Verification items for the finished model (mm, model axes). Face numbers are marked on the shaded views. Give positions to 0.01 mm unless a question says otherwise; leave off trailing zeros. Loops run counter-clockwise (first coordinate to the right, second up) from the corner with the lowest first, then second, coordinate; pieces in that order, holes last. Notation, with made-up numbers: M 70.5,18.5 L 115.5,18.5 A25 ccw 115.5,36.5 Z; hole C -19,53 d9. An arc over 180 degrees is marked long. Use CSV: the item, a comma, the result in double quotes.
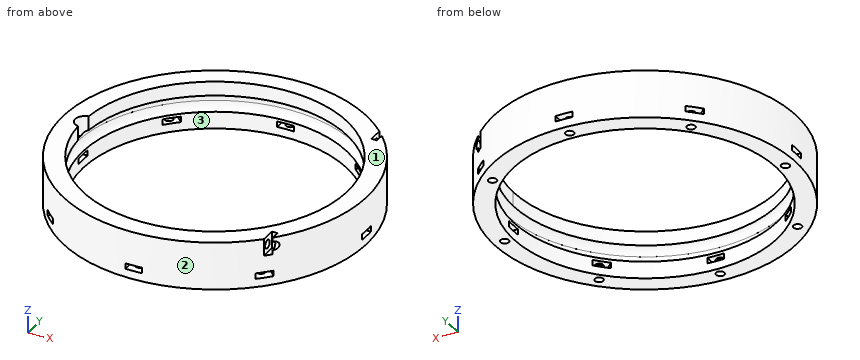
from build123d import *

# Parameters (mm, degrees)
BOX174_W                    = 2
BOX174_H                    = 6
BOX174_DEPTH                = 6
BOX175_W                    = 2
BOX175_H                    = 6
BOX175_DEPTH                = 6
BOX176_W                    = 2
BOX176_H                    = 6
BOX176_DEPTH                = 6
BOX173_W                    = 2
BOX173_H                    = 6
BOX173_DEPTH                = 6
CYLINDER397_R               = 1.5
CYLINDER397_DEPTH           = 100
CYLINDER398_R               = 1.5
CYLINDER398_DEPTH           = 100
CYLINDER395_R               = 1.5
CYLINDER395_DEPTH           = 100
CYLINDER396_R               = 1.5
CYLINDER396_DEPTH           = 100
CYLINDER375_R               = 1.5
CYLINDER375_DEPTH           = 50
CYLINDER375_PLACEMENT_ANGLE = 45
CYLINDER376_R               = 1.5
CYLINDER376_DEPTH           = 50
CYLINDER377_R               = 1.5
CYLINDER377_DEPTH           = 50
CYLINDER377_PLACEMENT_ANGLE = 135
CYLINDER378_R               = 1.5
CYLINDER378_DEPTH           = 50
CYLINDER379_R               = 1.5
CYLINDER379_DEPTH           = 50
CYLINDER379_PLACEMENT_ANGLE = 225
CYLINDER380_R               = 1.5
CYLINDER380_DEPTH           = 50
CYLINDER381_R               = 1.5
CYLINDER381_DEPTH           = 50
CYLINDER381_PLACEMENT_ANGLE = 45
CYLINDER374_R               = 1.5
CYLINDER374_DEPTH           = 50
BOX158_W                    = 8
BOX158_H                    = 6
BOX158_DEPTH                = 2
BOX158_PLACEMENT_ANGLE      = 45
BOX159_W                    = 8
BOX159_H                    = 6
BOX159_DEPTH                = 2
BOX160_W                    = 8
BOX160_H                    = 6
BOX160_DEPTH                = 2
BOX160_PLACEMENT_ANGLE      = 135
BOX161_W                    = 8
BOX161_H                    = 6
BOX161_DEPTH                = 2
BOX162_W                    = 8
BOX162_H                    = 6
BOX162_DEPTH                = 2
BOX162_PLACEMENT_ANGLE      = 225
BOX163_W                    = 8
BOX163_H                    = 6
BOX163_DEPTH                = 2
BOX164_W                    = 8
BOX164_H                    = 6
BOX164_DEPTH                = 2
BOX164_PLACEMENT_ANGLE      = 45
BOX157_W                    = 8
BOX157_H                    = 6
BOX157_DEPTH                = 2
CYLINDER006_R               = 3.5
CYLINDER006_DEPTH           = 10
TORUS004_R                  = 3.1
TUBE002_R                   = 54
TUBE002_R_2                 = 47
TUBE002_DEPTH               = 17


with BuildPart() as krychle174:
    # Box174 → Box174 (new body)
    with BuildSketch(Plane(origin=(32, -54, 22), x_dir=(1, 0, 0), z_dir=(0, 0, 1))):
        with Locations((1, 3)):
            Rectangle(BOX174_W, BOX174_H)
    extrude(amount=BOX174_DEPTH)


with BuildPart() as krychle175:
    # Box175 → Box175 (new body)
    with BuildSketch(Plane(origin=(38, 33, 31), x_dir=(1, 0, 0), z_dir=(0, 0, 1))):
        with Locations((1, 3)):
            Rectangle(BOX175_W, BOX175_H)
    extrude(amount=BOX175_DEPTH)


with BuildPart() as krychle176:
    # Box176 → Box176 (new body)
    with BuildSketch(Plane(origin=(38, -39, 31), x_dir=(1, 0, 0), z_dir=(0, 0, 1))):
        with Locations((1, 3)):
            Rectangle(BOX176_W, BOX176_H)
    extrude(amount=BOX176_DEPTH)


with BuildPart() as compound302:
    # Box173 → Box173 (new body)
    with BuildSketch(Plane(origin=(32, 48, 22), x_dir=(1, 0, 0), z_dir=(0, 0, 1))):
        with Locations((1, 3)):
            Rectangle(BOX173_W, BOX173_H)
    extrude(amount=BOX173_DEPTH)

    # Compound302: union Krychle174, Krychle175, Krychle176
    add(krychle174.part)
    add(krychle175.part)
    add(krychle176.part)


with BuildPart() as obj1:
    # Cylinder397 → Cylinder397 (new body)
    with BuildSketch(Plane(origin=(24, -51, 25), x_dir=(0, 0, -1), z_dir=(1, 0, 0))):
        Circle(CYLINDER397_R)
    extrude(amount=CYLINDER397_DEPTH)


with BuildPart() as obj2:
    # Cylinder398 → Cylinder398 (new body)
    with BuildSketch(Plane(origin=(34, 36, 34), x_dir=(0, 0, -1), z_dir=(1, 0, 0))):
        Circle(CYLINDER398_R)
    extrude(amount=CYLINDER398_DEPTH)


with BuildPart() as obj3:
    # Cylinder395 → Cylinder395 (new body)
    with BuildSketch(Plane(origin=(34, -36, 34), x_dir=(0, 0, -1), z_dir=(1, 0, 0))):
        Circle(CYLINDER395_R)
    extrude(amount=CYLINDER395_DEPTH)


with BuildPart() as compound303:
    # Cylinder396 → Cylinder396 (new body)
    with BuildSketch(Plane(origin=(24, 51, 25), x_dir=(0, 0, -1), z_dir=(1, 0, 0))):
        Circle(CYLINDER396_R)
    extrude(amount=CYLINDER396_DEPTH)

    # Compound303: union obj1, obj2, obj3
    add(obj1.part)
    add(obj2.part)
    add(obj3.part)


with BuildPart() as obj4:
    # Cylinder375 → Cylinder375 (new body)
    with BuildSketch(Plane.XY):
        Circle(CYLINDER375_R)
    extrude(amount=CYLINDER375_DEPTH)


with BuildPart() as obj4_1:
    # Cylinder375 placement: moved
    add(obj4.part.moved(Location((35.355339, 35.355339, -15))).rotate(Axis((35.355339, 35.355339, -15), (0, 0, 1)), CYLINDER375_PLACEMENT_ANGLE))


with BuildPart() as obj5:
    # Cylinder376 → Cylinder376 (new body)
    with BuildSketch(Plane(origin=(0, 50, -15), x_dir=(0, 1, 0), z_dir=(0, 0, 1))):
        Circle(CYLINDER376_R)
    extrude(amount=CYLINDER376_DEPTH)


with BuildPart() as obj6:
    # Cylinder377 → Cylinder377 (new body)
    with BuildSketch(Plane.XY):
        Circle(CYLINDER377_R)
    extrude(amount=CYLINDER377_DEPTH)


with BuildPart() as obj6_1:
    # Cylinder377 placement: moved
    add(obj6.part.moved(Location((-35.355339, 35.355339, -15))).rotate(Axis((-35.355339, 35.355339, -15), (0, 0, 1)), CYLINDER377_PLACEMENT_ANGLE))


with BuildPart() as obj7:
    # Cylinder378 → Cylinder378 (new body)
    with BuildSketch(Plane(origin=(-50, 0, -15), x_dir=(-1, 0, 0), z_dir=(0, 0, 1))):
        Circle(CYLINDER378_R)
    extrude(amount=CYLINDER378_DEPTH)


with BuildPart() as obj8:
    # Cylinder379 → Cylinder379 (new body)
    with BuildSketch(Plane.XY):
        Circle(CYLINDER379_R)
    extrude(amount=CYLINDER379_DEPTH)


with BuildPart() as obj8_1:
    # Cylinder379 placement: moved
    add(obj8.part.moved(Location((-35.355339, -35.355339, -15))).rotate(Axis((-35.355339, -35.355339, -15), (0, 0, 1)), CYLINDER379_PLACEMENT_ANGLE))


with BuildPart() as obj9:
    # Cylinder380 → Cylinder380 (new body)
    with BuildSketch(Plane(origin=(0, -50, -15), x_dir=(0, -1, 0), z_dir=(0, 0, 1))):
        Circle(CYLINDER380_R)
    extrude(amount=CYLINDER380_DEPTH)


with BuildPart() as obj10:
    # Cylinder381 → Cylinder381 (new body)
    with BuildSketch(Plane.XY):
        Circle(CYLINDER381_R)
    extrude(amount=CYLINDER381_DEPTH)


with BuildPart() as obj10_1:
    # Cylinder381 placement: moved
    add(obj10.part.moved(Location((35.355339, -35.355339, -15))).rotate(Axis((35.355339, -35.355339, -15), (0, 0, -1)), CYLINDER381_PLACEMENT_ANGLE))


with BuildPart() as compound298:
    # Cylinder374 → Cylinder374 (new body)
    with BuildSketch(Plane(origin=(50, 0, -15), x_dir=(1, 0, 0), z_dir=(0, 0, 1))):
        Circle(CYLINDER374_R)
    extrude(amount=CYLINDER374_DEPTH)

    # Compound298: union obj4, obj5, obj6, obj7, obj8, obj9, obj10
    add(obj4_1.part)
    add(obj5.part)
    add(obj6_1.part)
    add(obj7.part)
    add(obj8_1.part)
    add(obj9.part)
    add(obj10_1.part)


with BuildPart() as compound298_1:
    # Compound298 placement: moved
    add(compound298.part.moved(Location((0, 0, -9))))


with BuildPart() as krychle158:
    # Box158 → Box158 (new body)
    with BuildSketch(Plane.XY):
        with Locations((4, 3)):
            Rectangle(BOX158_W, BOX158_H)
    extrude(amount=BOX158_DEPTH)


with BuildPart() as krychle158_1:
    # Box158 placement: moved
    add(krychle158.part.moved(Location((34.648232, 30.405592, 23))).rotate(Axis((34.648232, 30.405592, 23), (0, 0, 1)), BOX158_PLACEMENT_ANGLE))


with BuildPart() as krychle159:
    # Box159 → Box159 (new body)
    with BuildSketch(Plane(origin=(3, 46, 23), x_dir=(0, 1, 0), z_dir=(0, 0, 1))):
        with Locations((4, 3)):
            Rectangle(BOX159_W, BOX159_H)
    extrude(amount=BOX159_DEPTH)


with BuildPart() as krychle160:
    # Box160 → Box160 (new body)
    with BuildSketch(Plane.XY):
        with Locations((4, 3)):
            Rectangle(BOX160_W, BOX160_H)
    extrude(amount=BOX160_DEPTH)


with BuildPart() as krychle160_1:
    # Box160 placement: moved
    add(krychle160.part.moved(Location((-30.405592, 34.648232, 23))).rotate(Axis((-30.405592, 34.648232, 23), (0, 0, 1)), BOX160_PLACEMENT_ANGLE))


with BuildPart() as krychle161:
    # Box161 → Box161 (new body)
    with BuildSketch(Plane(origin=(-46, 3, 23), x_dir=(-1, 0, 0), z_dir=(0, 0, 1))):
        with Locations((4, 3)):
            Rectangle(BOX161_W, BOX161_H)
    extrude(amount=BOX161_DEPTH)


with BuildPart() as krychle162:
    # Box162 → Box162 (new body)
    with BuildSketch(Plane.XY):
        with Locations((4, 3)):
            Rectangle(BOX162_W, BOX162_H)
    extrude(amount=BOX162_DEPTH)


with BuildPart() as krychle162_1:
    # Box162 placement: moved
    add(krychle162.part.moved(Location((-34.648232, -30.405592, 23))).rotate(Axis((-34.648232, -30.405592, 23), (0, 0, 1)), BOX162_PLACEMENT_ANGLE))


with BuildPart() as krychle163:
    # Box163 → Box163 (new body)
    with BuildSketch(Plane(origin=(-3, -46, 23), x_dir=(0, -1, 0), z_dir=(0, 0, 1))):
        with Locations((4, 3)):
            Rectangle(BOX163_W, BOX163_H)
    extrude(amount=BOX163_DEPTH)


with BuildPart() as krychle164:
    # Box164 → Box164 (new body)
    with BuildSketch(Plane.XY):
        with Locations((4, 3)):
            Rectangle(BOX164_W, BOX164_H)
    extrude(amount=BOX164_DEPTH)


with BuildPart() as krychle164_1:
    # Box164 placement: moved
    add(krychle164.part.moved(Location((30.405592, -34.648232, 23))).rotate(Axis((30.405592, -34.648232, 23), (0, 0, -1)), BOX164_PLACEMENT_ANGLE))


with BuildPart() as compound297:
    # Box157 → Box157 (new body)
    with BuildSketch(Plane(origin=(46, -3, 23), x_dir=(1, 0, 0), z_dir=(0, 0, 1))):
        with Locations((4, 3)):
            Rectangle(BOX157_W, BOX157_H)
    extrude(amount=BOX157_DEPTH)

    # Compound297: union Krychle158, Krychle159, Krychle160, Krychle161, Krychle162, Krychle163, Krychle164
    add(krychle158_1.part)
    add(krychle159.part)
    add(krychle160_1.part)
    add(krychle161.part)
    add(krychle162_1.part)
    add(krychle163.part)
    add(krychle164_1.part)


with BuildPart() as obj11:
    # Cylinder006 → Cylinder006 (new body)
    with BuildSketch(Plane(origin=(-46.3, 0, 30), x_dir=(1, 0, 0), z_dir=(0, 0, 1))):
        Circle(CYLINDER006_R)
    extrude(amount=CYLINDER006_DEPTH)


with BuildPart() as obj12:
    # Torus004 → Torus004 (revolve)
    with BuildSketch(Plane(origin=(0, 0, 29), x_dir=(1, 0, 0), z_dir=(0, -1, 0))):
        with Locations((46, 0)):
            Circle(TORUS004_R)
    revolve(axis=Axis((0, 0, 29), (0, 0, 1)))


with BuildPart() as cut160:
    # Tube002 → Tube002 (new body)
    with BuildSketch(Plane.XY.offset(20)):
        Circle(TUBE002_R)
        Circle(TUBE002_R_2, mode=Mode.SUBTRACT)
    extrude(amount=TUBE002_DEPTH)

    # Cut009: cut obj12
    add(obj12.part, mode=Mode.SUBTRACT)

    # Cut010: cut obj11
    add(obj11.part, mode=Mode.SUBTRACT)

    # Cut151: cut Compound297
    add(compound297.part, mode=Mode.SUBTRACT)

    # Cut152: cut Compound298
    add(compound298_1.part, mode=Mode.SUBTRACT)

    # Cut159: cut Compound303
    add(compound303.part, mode=Mode.SUBTRACT)

    # Cut160: cut Compound302
    add(compound302.part, mode=Mode.SUBTRACT)


solid = cut160.part
(1) Section check B-B on z = 27.75. Record the cut outline in (x, y).
Calculated:
outline,"C 0,0 d108; hole C 0,0 d97.67"
(2) Mould release check, pull along X, two halves, no side actions. Record for the marked faces 1, 2 and 3: released by +X, released by -X, zero draft, split by the parting line, or undercut.
Calculated:
face 1,"zero draft"
face 2,"split by the parting line"
face 3,"undercut"
(3) Scan lines: L1, parallel to Z at x = 35.2, y = -36; L2, parallel to X at y = -33.5, z = 34.25; L3, parallel to X at y = -50, z = 21.3. Record each from-to range of solid material in increasing order. Write a range as from..to.
Calculated:
L1,"z = 26..32.5, 35.5..37"
L2,"x = -42.35..-32.97, 32.97..38, 40..42.35"
L3,"x = -20.4..-1.5, 1.5..20.4"
(4) Section check A-A on z = 34. Record the cut outline in (x, y).
Calculated:
outline,"M 34,-37.5 L 34,-34.5 L 38,-34.5 L 38,-33 L 40,-33 L 40,-34.5 L 41.54,-34.5 A54 ccw 41.54,34.5 L 40,34.5 L 40,33 L 38,33 L 38,34.5 L 34,34.5 L 34,37.5 L 38,37.5 L 38,38.37 A54 ccw long 38,-38.37 L 38,-37.5 Z; hole M -46.87,-3.45 A47 ccw long -46.87,3.45 A3.5 ccw Z"
(5) Depth check by flat-ended pin: pin 1 Ø2 at (x, z) = (-13, 32) entering from +Y; pin 2 Ø1 at (y, z) = (9.5, 28) entering from -X; pin 3 Ø5 at (x, y) = (-35.36, -35.36) entering from -Z; pin 4 Ø3 at (y, z) = (38, 26) entering from -X. Enter the tip coordinate at first touch or a pass-through.
Calculated:
pin 1,"stops at y = 52.65"
pin 2,"stops at x = -53.24"
pin 3,"stops at z = 20"
pin 4,"stops at x = -39.8"
